Read the model definition and answer for the solid it produces. Units are mm, in the model's axes. Give positions to 0.01 mm unless a question says otherwise; leave off trailing zeros. Loops run counter-clockwise (first coordinate to the right, second up) from the corner with the lowest first, then second, coordinate; pieces in that order, holes last. Notation, with made-up numbers: (11, 82.5) -> (36, 82.5) arc R5 ccw to (36, 91.5) -> close; hole circle Ø1 at (64.25, -12.5). An arc over 180 degrees is marked (long way). Return JSON: item names as keys, results as strings. Group by question number.
from build123d import *

# Parameters (mm, degrees)
SKETCH1_R           = 1.5
SKETCH1_R_2         = 1.25
BOSS_EXTRUDE1_DEPTH = 2.5


with BuildPart() as part:
    # Sketch1 → Boss-Extrude1 (new body)
    with BuildSketch(Plane(origin=(0, 0, 0), x_dir=(0, 0, -1), z_dir=(1, 0, 0))):
        with BuildLine():
            Line((-7, 0), (-7, 60))
            ThreePointArc((-7, 60), (0, 67), (7, 60))
            Line((7, 60), (7, 0))
            ThreePointArc((7, 0), (0, -7), (-7, 0))
        make_face()
        Circle(SKETCH1_R, mode=Mode.SUBTRACT)
        with Locations((0, 60)):
            Circle(SKETCH1_R, mode=Mode.SUBTRACT)
        with Locations((0, 45)):
            Circle(SKETCH1_R_2, mode=Mode.SUBTRACT)
        with Locations((0, 40)):
            Circle(SKETCH1_R_2, mode=Mode.SUBTRACT)
        with Locations((0, 35)):
            Circle(SKETCH1_R_2, mode=Mode.SUBTRACT)
        with Locations((0, 30)):
            Circle(SKETCH1_R_2, mode=Mode.SUBTRACT)
    extrude(amount=BOSS_EXTRUDE1_DEPTH)


solid = part.part
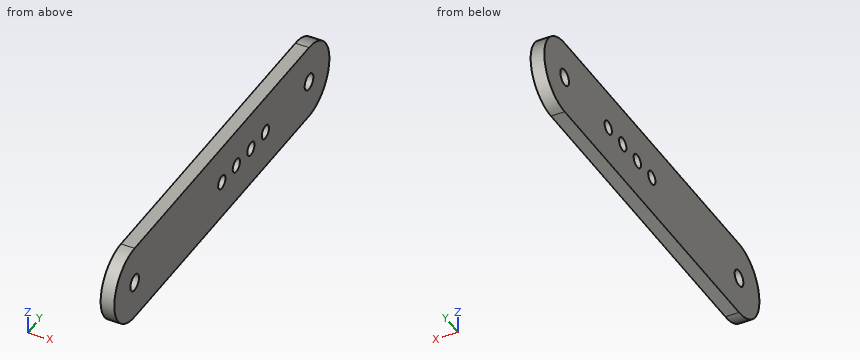
1. Section D-D on z = -4 is taken. Determine the outline of the cut face in (x, y), then the cut area to 3 significant figures.
2. Straight lines are drawn through the part: line 1 (Z direction, x = 2, y = -1); line 2 (Y direction, x = 2.05, z = -2.5); line 3 (Y direction, x = 0.45, z = -3). For each, find the intervals that lie inside material, in ascending order. Write a range as from..to.
3. A flat-ended cylindrical pin translates along its axis: pin 1 Ø1.8 at (y, z) = (60, 0) entering from -X. Find the tip coordinate at first contact, or state that the pin passes through.
4. Section B-B on x = 1.9 is taken. Determine the outline of the cut face in (y, z), then the cut area to 3 significant figures.
5. Section A-A on y = 40 is taken. Determine the outline of the cut face in (x, z), then the cut area to 4 significant figures.
6. Section C-C on z = 0 is taken. Determine the outline of the cut face in (x, y).
Completed:
{
 "1": {"outline": "(0, -5.74) -> (2.5, -5.74) -> (2.5, 65.74) -> (0, 65.74) -> close", "area": "179 mm²"},
 "2": {"line 1": "z = -6.93..-1.12, 1.12..6.93", "line 2": "y = -6.54..66.54", "line 3": "y = -6.32..66.32"},
 "3": {"pin 1": "passes through"},
 "4": {"outline": "(0, -7) -> (60, -7) arc R7 ccw to (60, 7) -> (0, 7) arc R7 ccw to start; hole circle Ø3 at (0, 0); hole circle Ø2.5 at (30, 0); hole circle Ø2.5 at (35, 0); hole circle Ø2.5 at (40, 0); hole circle Ø2.5 at (45, 0); hole circle Ø3 at (60, 0)", "area": "960 mm²"},
 "5": {"outline": "(0, -7) -> (2.5, -7) -> (2.5, -1.25) -> (0, -1.25) -> close; (0, 1.25) -> (2.5, 1.25) -> (2.5, 7) -> (0, 7) -> close", "area": "28.75 mm²"},
 "6": {"outline": "(0, -7) -> (2.5, -7) -> (2.5, -1.5) -> (0, -1.5) -> close; (0, 1.5) -> (2.5, 1.5) -> (2.5, 28.75) -> (0, 28.75) -> close; (0, 31.25) -> (2.5, 31.25) -> (2.5, 33.75) -> (0, 33.75) -> close; (0, 36.25) -> (2.5, 36.25) -> (2.5, 38.75) -> (0, 38.75) -> close; (0, 41.25) -> (2.5, 41.25) -> (2.5, 43.75) -> (0, 43.75) -> close; (0, 46.25) -> (2.5, 46.25) -> (2.5, 58.5) -> (0, 58.5) -> close; (0, 61.5) -> (2.5, 61.5) -> (2.5, 67) -> (0, 67) -> close"}
}
